Part model, mm, in its own coordinate system. A direction names the side the tool comes from. Coordinates: 2 decimals unless noted, no trailing zeros. Loops run counter-clockwise (first coordinate to the right, second up) from the corner with the lowest first, then second, coordinate; pieces in that order, holes last. Notation, with made-up numbers: (79, -17.5) - (134, -17.5) arc R23 cw to (134, -6.5) - close; hole circle Ø6 at (57, 50). An arc over 180 degrees is marked (long way). Use a Markdown table: item, result. Add a question column.
1) Tool access for faces 4 (the face through (11.5, 8, 0)), 5 (the face through (-11.5, 21, 0)), 6 (the face through (-11.5, 8, 0)), 7 (the face through (11.496, 25.272, 0.229)): list every direction of +Z, -Z, +X, -X, +Y, -Y with a clear straight run to the whole face (end or side of a thin tool).
2) Band-saw the part on B-B (x = -0.6). Give the cut face in (y, z), plus the area to 3 significant figures.
3) Band-saw the part on C-C (z = -4.5). Give the cut face in (x, y), plus the area to 3 significant figures.
4) Probe probe 1 along X at (y, z) = (17.65, 0); probe 2 along X at (y, z) = (17.5, -0.5); probe 3 along Z at (x, y) = (14, 18.05). List the from-to ranges inside material, lowest first. Write a range as [from, to].
5) Pull direction X, two halves, no side cores. Call faces 1 (the face through (16.5, 18, 0)), 2 (the face through (-12.76, 17.57, -0.16)), 3 (the face through (-16.5, 18, 0)): +X half, -X half, draft (parallel to the pull), parting line (faces both ways), or undercut.
6) Band-saw the part on D-D (y = 8.75). Give the cut face in (x, z).
7) Drop flat-ended pins along their axis: P1, Ø2, axis at y = 20, z = 3, coming from the -X side; P2, Ø3, axis at x = -7.5, z = 0.5, coming from the -Y side; P3, Ø3.5, axis at x = -6, z = -2.5, coming from the +Y side; P4, Ø2.5, axis at x = -14.5, z = -1, coming from the -Y side. Give the stop position or say it passes through.
8) Band-saw the part on A-A (x = 14). Give the cut face in (y, z).
from build123d import *

# Parameters (mm, degrees)
SKETCH1_W           = 23
SKETCH1_H           = 12.2
BOSS_EXTRUDE1_DEPTH = 23.3
BOSS_EXTRUDE2_START = -4.5
SKETCH2_W           = 5
SKETCH2_H           = 12.2
SKETCH2_R           = 1.25
BOSS_EXTRUDE2_DEPTH = 2.5
SKETCH3_R           = 2.15
BOSS_EXTRUDE3_DEPTH = 4
BOSS_EXTRUDE4_START = 4
SKETCH3_4_R         = 2.15
BOSS_EXTRUDE4_DEPTH = 2.5


with BuildPart() as part:
    # Sketch1 → Boss-Extrude1 (new body)
    with BuildSketch(Plane(origin=(0, 0, 0), x_dir=(1, 0, 0), z_dir=(0, 1, 0))):
        Rectangle(SKETCH1_W, SKETCH1_H)
    extrude(amount=BOSS_EXTRUDE1_DEPTH)

    # Sketch2 → Boss-Extrude2 (add)
    # profile 1 of 2: a face of its own
    with BuildSketch(Plane(origin=(0, 23.3, 0), x_dir=(1, 0, 0), z_dir=(0, 1, 0)).offset(BOSS_EXTRUDE2_START)):
        with Locations((-14, 0)):
            Rectangle(SKETCH2_W, SKETCH2_H)
        with Locations(Location((-14, 0, 0), (0, 0, 270))):
            Circle(SKETCH2_R, mode=Mode.SUBTRACT)
    # profile 2 of 2: a face of its own
    with BuildSketch(Plane(origin=(0, 23.3, 0), x_dir=(1, 0, 0), z_dir=(0, 1, 0)).offset(BOSS_EXTRUDE2_START)):
        with Locations((14, 0)):
            Rectangle(SKETCH2_W, SKETCH2_H)
        with Locations(Location((14, 0, 0), (0, 0, 90))):
            Circle(SKETCH2_R, mode=Mode.SUBTRACT)
    extrude(amount=-BOSS_EXTRUDE2_DEPTH)

    # Sketch3 → Boss-Extrude3 (add)
    # profile 1 of 2: a face of its own
    with BuildSketch(Plane(origin=(0, 23.3, 0), x_dir=(1, 0, 0), z_dir=(0, 1, 0))):
        with BuildLine():
            ThreePointArc((-0.070625, -2.698566677), (11.5, 0), (-0.070625, 2.698566677))
            ThreePointArc((-0.070625, 2.698566677), (-3.35, 0), (-0.070625, -2.698566677))
        make_face()
        with Locations((5.4, 0)):
            Circle(SKETCH3_R, mode=Mode.SUBTRACT)
    # profile 2 of 2: a face of its own
    with BuildSketch(Plane(origin=(0, 23.3, 0), x_dir=(1, 0, 0), z_dir=(0, 1, 0))):
        with Locations((5.4, 0)):
            Circle(SKETCH3_R)
    extrude(amount=BOSS_EXTRUDE3_DEPTH)

    # Sketch3<4> → Boss-Extrude4 (add)
    with BuildSketch(Plane(origin=(0, 23.3, 0), x_dir=(1, 0, 0), z_dir=(0, 1, 0)).offset(BOSS_EXTRUDE4_START)):
        with Locations(Location((5.4, 0, 0), (0, 0, 270))):
            Circle(SKETCH3_4_R)
    extrude(amount=BOSS_EXTRUDE4_DEPTH)


solid = part.part
Answer block:
| question | item | result |
|---|---|---|
| 1 | face 4 | +Z, -Z, +X, -Y |
| 1 | face 5 | +Z, -Z, -X, +Y |
| 1 | face 6 | +Z, -Z, -X, -Y |
| 1 | face 7 | +Y |
| 2 | outline | (0, -6.1) - (23.3, -6.1) - (23.3, -2.75) - (27.3, -2.75) - (27.3, 2.75) - (23.3, 2.75) - (23.3, 6.1) - (0, 6.1) - close |
| 2 | area | 306 mm2 |
| 3 | outline | (-16.5, 16.3) - (-11.5, 16.3) - (-11.5, 0) - (11.5, 0) - (11.5, 16.3) - (16.5, 16.3) - (16.5, 18.8) - (11.5, 18.8) - (11.5, 23.3) - (9.52, 23.3) - (9.52, 27.3) - (1.28, 27.3) - (1.28, 23.3) - (-11.5, 23.3) - (-11.5, 18.8) - (-16.5, 18.8) - close |
| 3 | area | 594 mm2 |
| 4 | probe 1 | [-16.5, -15.25], [-12.75, 12.75], [15.25, 16.5] |
| 4 | probe 2 | [-16.5, -15.15], [-12.85, 12.85], [15.15, 16.5] |
| 4 | probe 3 | [-6.1, -1.25], [1.25, 6.1] |
| 5 | face 1 | +X half |
| 5 | face 2 | undercut |
| 5 | face 3 | -X half |
| 6 | outline | (-11.5, -6.1) - (11.5, -6.1) - (11.5, 6.1) - (-11.5, 6.1) - close |
| 7 | P1 | x = -11.5 |
| 7 | P2 | y = 0 |
| 7 | P3 | y = 23.3 |
| 7 | P4 | y = 16.3 |
| 8 | outline | (16.3, -6.1) - (18.8, -6.1) - (18.8, -1.25) - (16.3, -1.25) - close; (16.3, 1.25) - (18.8, 1.25) - (18.8, 6.1) - (16.3, 6.1) - close |
